Input: dimensioned drawing with shaded views. Units: mm. Origin: part minimum x, y, z. A direction names the side the tool comes from. Round coordinates to 2 decimals unless told otherwise and drop trailing zeros. Write each loop counter-clockwise with the first axis right and the second up, starting at its lowest first coordinate (ties: lowest second). Pieces come first, ordered by that corner, then holes. Notation, with made-up numbers: M -21,-22 L 34,-22 A33 ccw 34,10 Z; hole C 26.25,-37 d4. An arc over 180 degrees is marked long. Answer as CSV lines item,"result". Start each with the question number.
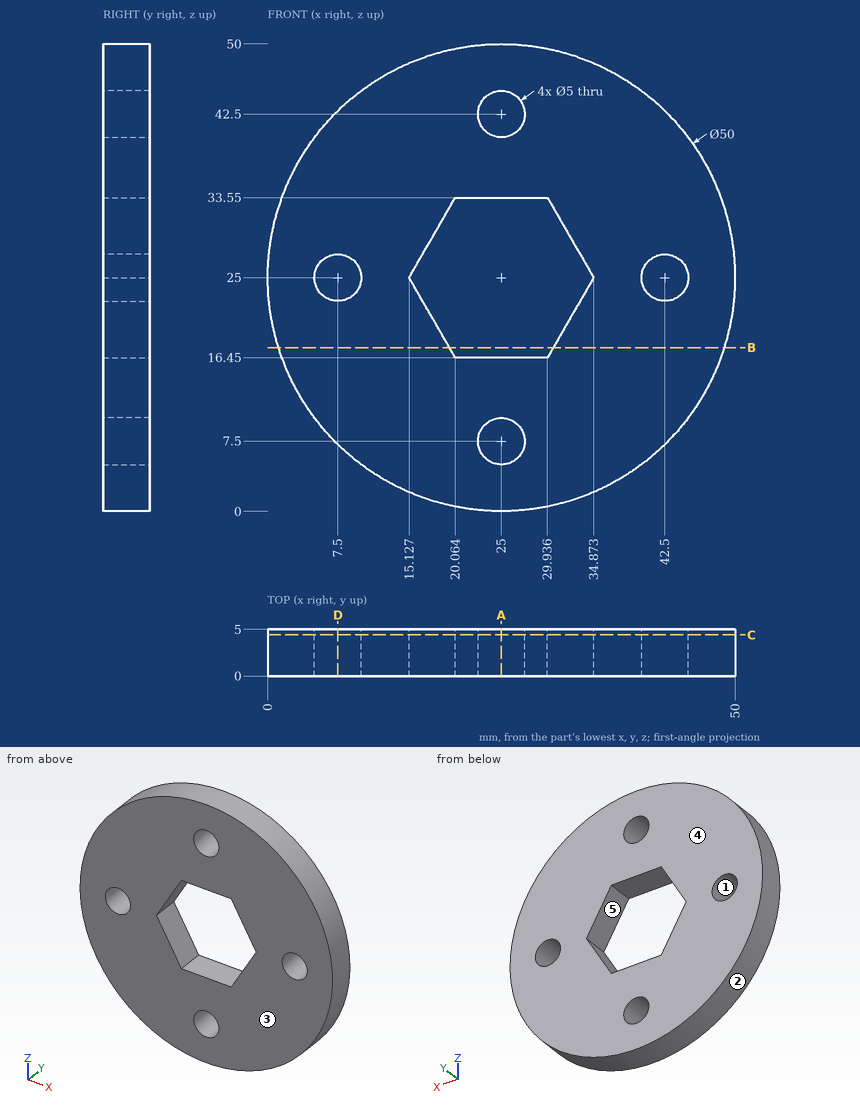
Item 1: Cut plane A-A, the plane x = 25. Return loops of the section in (y, z).
Item 2: Pin query (flat end, axial travel): pin 1 Ø1 at (x, y) = (36.5, 1.5) entering from +Z; pin 2 Ø6 at (x, z) = (42.5, 25) entering from -Y; pin 3 Ø1 at (x, y) = (14.5, 2.5) entering from +Z; pin 4 Ø1.5 at (y, z) = (4, 35.5) entering from +X. Return the tip coordinate at first contact, or that it passes through.
Item 3: Cut plane B-B, the plane z = 17.5. Return loops of the section in (x, y).
Item 4: Draft query along Z for the marked faces 1, 2 and 3. Return one class per face: +Z half, -Z half, draft (parallel to the pull), parting line (faces both ways), or undercut.
Item 5: Line query: line 1 (X direction, y = 2.3, z = 25); line 2 (Z direction, x = 26, y = 0.8); line 3 (X direction, y = 2.55, z = 42.5) (1 decimal). Output: solid intervals per line, ascending. Write a range as [from, to].
Item 6: Access query for the marked faces 4 and 5. Directions: +Z, -Z, +X, -X, +Y, -Y. A direction counts if a zero-diameter tool reaches every point of the face in a straight line with its end or side. Return the directions, or none.
Item 7: Cut plane D-D, the plane x = 7.5. Return loops of the section in (y, z).
Item 8: Cut plane C-C, the plane y = 4.4. Return loops of the section in (x, z).
Results list:
1,outline,"M 0,0 L 5,0 L 5,5 L 0,5 Z; M 0,10 L 5,10 L 5,16.45 L 0,16.45 Z; M 0,33.55 L 5,33.55 L 5,40 L 0,40 Z; M 0,45 L 5,45 L 5,50 L 0,50 Z"
2,pin 1,"z = 47.45"
2,pin 2,"y = 0"
2,pin 3,"z = 47.91"
2,pin 4,"x = 48.02"
3,outline,"M 1.15,0 L 19.46,0 L 19.46,5 L 1.15,5 Z; M 30.54,0 L 48.85,0 L 48.85,5 L 30.54,5 Z"
4,face 1,"undercut"
4,face 2,"parting line"
4,face 3,"draft"
5,line 1,"[0, 5], [10, 15.13], [34.87, 40], [45, 50]"
5,line 2,"[0.02, 5.21], [9.79, 16.45], [33.55, 40.21], [44.79, 49.98]"
5,line 3,"[7.1, 22.5], [27.5, 42.9]"
6,face 4,"+Z, -Z, +X, -X, +Y"
6,face 5,"+Y, -Y"
7,outline,"M 0,7.15 L 5,7.15 L 5,22.5 L 0,22.5 Z; M 0,27.5 L 5,27.5 L 5,42.85 L 0,42.85 Z"
8,outline,"C 25,25 d50; hole C 7.5,25 d5; hole M 15.13,25 L 20.06,16.45 L 29.94,16.45 L 34.87,25 L 29.94,33.55 L 20.06,33.55 Z; hole C 25,7.5 d5; hole C 25,42.5 d5; hole C 42.5,25 d5"
